from build123d import *

# Parameters (mm, degrees)
SKETCH2_W           = 18.7
SKETCH2_H           = 20
BOSS_EXTRUDE1_DEPTH = 25.4
SKETCH3_W           = 6.35
SKETCH3_H           = 7.3
SKETCH3_H_2         = 3.175
CUT_EXTRUDE1_DEPTH  = 21
SKETCH5_W           = 3.175
SKETCH5_H           = 25.4
BOSS_EXTRUDE2_DEPTH = 20
SKETCH6_W           = 10
SKETCH6_H           = 10.125
CUT_EXTRUDE2_DEPTH  = 16.825
SKETCH7_W           = 3
SKETCH7_H           = 3.5
CUT_EXTRUDE3_DEPTH  = 10
SKETCH8_W           = 22
SKETCH8_H           = 10.125
CUT_EXTRUDE4_DEPTH  = 19
SKETCH9_W           = 2.175
SKETCH9_H           = 14.925
BOSS_EXTRUDE3_DEPTH = 25.05


with BuildPart() as part:
    # Sketch2 → Boss-Extrude1 (new body)
    with BuildSketch(Plane(origin=(0, 0, 0), x_dir=(1, 0, 0), z_dir=(0, 1, 0))):
        Rectangle(SKETCH2_W, SKETCH2_H)
    extrude(amount=BOSS_EXTRUDE1_DEPTH)

    # Sketch3 → Cut-Extrude1 (cut, through all)
    with BuildSketch(Plane(origin=(0, 0, -10), x_dir=(-1, 0, 0), z_dir=(0, 0, -1))):
        with Locations((0, 21.75)):
            Rectangle(SKETCH3_W, SKETCH3_H)
        with Locations((0, 16.5125)):
            Rectangle(SKETCH3_W, SKETCH3_H_2)
    extrude(amount=-CUT_EXTRUDE1_DEPTH, mode=Mode.SUBTRACT)

    # Sketch5 → Boss-Extrude2 (add)
    with BuildSketch(Plane(origin=(0, 0, -10), x_dir=(-1, 0, 0), z_dir=(0, 0, -1))):
        with Locations((-10.9375, 12.7)):
            Rectangle(SKETCH5_W, SKETCH5_H)
        with Locations((10.9375, 12.7)):
            Rectangle(SKETCH5_W, SKETCH5_H)
    extrude(amount=-BOSS_EXTRUDE2_DEPTH)

    # Sketch6 → Cut-Extrude2 (cut)
    with BuildSketch(Plane(origin=(0, 0, -10), x_dir=(-1, 0, 0), z_dir=(0, 0, -1))):
        Polygon((5, 22.225), (5, 10.125), (5, 0), (9.35, 0), (9.35, 22.225), align=None)
        with Locations((0, 5.0625)):
            Rectangle(SKETCH6_W, SKETCH6_H)
        Polygon((-5, 22.225), (-9.35, 22.225), (-9.35, 0), (-5, 0), (-5, 10.125), align=None)
    extrude(amount=-CUT_EXTRUDE2_DEPTH, mode=Mode.SUBTRACT)

    # Sketch7 → Cut-Extrude3 (cut)
    with BuildSketch(Plane(origin=(5, 0, 0), x_dir=(0, 0, -1), z_dir=(1, 0, 0))):
        with Locations((-4.825, 19.725)):
            Rectangle(SKETCH7_W, SKETCH7_H)
    extrude(amount=-CUT_EXTRUDE3_DEPTH, mode=Mode.SUBTRACT)

    # Sketch8 → Cut-Extrude4 (cut)
    with BuildSketch(Plane(origin=(0, 0, -10), x_dir=(-1, 0, 0), z_dir=(0, 0, -1))):
        with Locations((0, 5.0625)):
            Rectangle(SKETCH8_W, SKETCH8_H)
    extrude(amount=-CUT_EXTRUDE4_DEPTH, mode=Mode.SUBTRACT)

    # Sketch9 → Boss-Extrude3 (add)
    with BuildSketch(Plane(origin=(12.525, 0, 0), x_dir=(0, 0, -1), z_dir=(1, 0, 0))):
        with Locations((-11.0875, 7.4625)):
            Rectangle(SKETCH9_W, SKETCH9_H)
    extrude(amount=-BOSS_EXTRUDE3_DEPTH)


solid = part.part
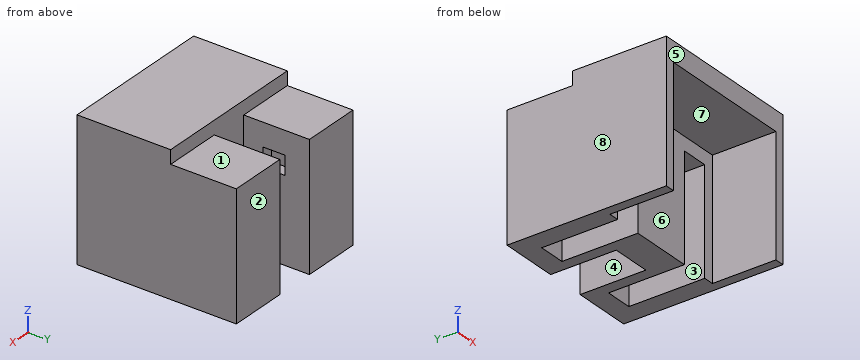
Model file for the job. Use its own axes, mm. Face numbers are marked on the shaded views. A direction names the side the tool comes from. Round coordinates to 2 decimals unless told otherwise and drop trailing zeros. Loops run counter-clockwise (first coordinate to the right, second up) from the corner with the lowest first, then second, coordinate; pieces in that order, holes last. Notation, with made-up numbers: (-22, -10) - (35, -10) arc R32 ccw to (35, 25) - close; hole circle Ø1 at (61, -21.75). An arc over 180 degrees is marked (long way). Write each question's results on one line, items separated by ' | '.
(1) Mould opens along X. For the marked faces 5, 6, 7 and 8 say: released by +X, released by -X, zero draft, split by the parting line, or undercut.
Answer below:
face 5: zero draft | face 6: undercut | face 7: undercut | face 8: released by -X
(2) Saw through at A-A, the plane y = 16. List the corners of the cut face in (x, z) (3 decimals), then the cut area to 3 significant figures.
Answer below:
outline: (-12.525, -10) - (-9.35, -10) - (-9.35, 6.825) - (-5, 6.825) - (-5, -10) - (-3.175, -10) - (-3.175, 10) - (-12.525, 10) - close; (3.175, -10) - (5, -10) - (5, 6.825) - (9.35, 6.825) - (9.35, -10) - (12.525, -10) - (12.525, 10) - (3.175, 10) - close | area: 228 mm^2
(3) Wall check: L1, parallel to X at y = 19.75, z = -2.25 (3 decimals); L2, parallel to X at y = 10.75, z = 4.5 (3 decimals); L3, parallel to X at y = 4, z = -7.5 (3 decimals). Give the ranges that are in metal, low to high.
Answer below:
L1: x = -12.525 to -9.35, -5 to -3.175, 3.175 to 5, 9.35 to 12.525 | L2: x = -12.525 to -9.35, -5 to 5, 9.35 to 12.525 | L3: x = -12.525 to -11, 11 to 12.525
(4) Pin check, flat tips, straight feed: pin 1 (1.3 mm diameter, centred on x = 7, y = 14, fed in from -Z) (3 decimals); pin 2 (5 mm diameter, centred on x = 8, z = 1, fed in from -Y) (3 decimals); pin 3 (3 mm diameter, centred on x = -7, y = 20, fed in from +Z). Stop position of each tip, or through.
Answer below:
pin 1: stops at z = 6.825 | pin 2: stops at y = 10.125 | pin 3: stops at z = 10
(5) Saw through at B-B, the plane z = 4. List the corners of the cut face in (x, y) (3 decimals).
Answer below:
outline: (-12.525, 0) - (-11, 0) - (-11, 10.125) - (-9.35, 10.125) - (-9.35, 22.225) - (-5, 22.225) - (-5, 21.475) - (-3.175, 21.475) - (-3.175, 25.4) - (-12.525, 25.4) - close; (-5, 10.125) - (5, 10.125) - (5, 17.975) - (3.175, 17.975) - (3.175, 14.925) - (-3.175, 14.925) - (-3.175, 17.975) - (-5, 17.975) - close; (3.175, 21.475) - (5, 21.475) - (5, 22.225) - (9.35, 22.225) - (9.35, 10.125) - (11, 10.125) - (11, 0) - (12.525, 0) - (12.525, 25.4) - (3.175, 25.4) - close
(6) 3-axis set-ups, long thin cutter, end or side, ignore diameter. For the marked faces 1, 2, 3 and 4: which of +Z, -Z, +X, -X, +Y, -Y reach the whole face in a straight line?
Answer below:
face 1: +Z, +X, -X, +Y | face 2: +Z, -Z, +X, -X, +Y | face 3: -Z, -Y | face 4: +Z, -Z, +Y
(7) Saw through at C-C, the plane x = 5.75. List the corners of the cut face in (y, z) (3 decimals).
Answer below:
outline: (0, 9) - (10.125, 9) - (10.125, 6.825) - (22.225, 6.825) - (22.225, -10) - (25.4, -10) - (25.4, 10) - (14.925, 10) - (14.925, 12.175) - (0, 12.175) - close
(8) Saw through at D-D, the plane z = -3. List the corners of the cut face in (x, y) (3 decimals), then the cut area to 3 significant figures.
Answer below:
outline: (-12.525, 0) - (-11, 0) - (-11, 10.125) - (-9.35, 10.125) - (-9.35, 22.225) - (-5, 22.225) - (-5, 10.125) - (5, 10.125) - (5, 22.225) - (9.35, 22.225) - (9.35, 10.125) - (11, 10.125) - (11, 0) - (12.525, 0) - (12.525, 25.4) - (3.175, 25.4) - (3.175, 14.925) - (-3.175, 14.925) - (-3.175, 25.4) - (-12.525, 25.4) - close | area: 242 mm^2
